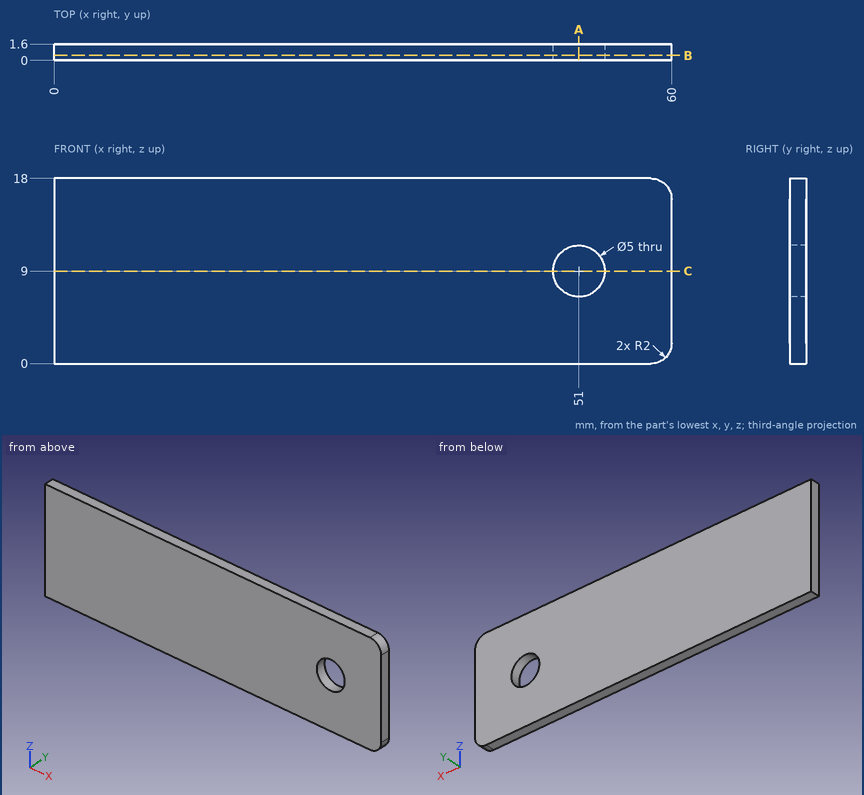
Can you work these out from the drawing? Everything is in mm from the part's minimum corner. Round coordinates to 2 decimals unless told otherwise and drop trailing zeros. Order: outer loops, then holes, each group sorted by start corner. A loop starts at its lowest first (then second) coordinate and runs counter-clockwise, first axis right, second up. Notation, with made-up numbers: (71, -25) -> (130, -25) arc R20 cw to (130, 9) -> close; hole circle Ø9 at (10, 71). An arc over 180 degrees is marked (long way). Return JSON: item names as keys, results as strings. Group by question number.
1. If we section it at B-B, the plane y = 0.5: Write out the boundary of the cut face in (x, z).
2. If we section it at A-A, the plane x = 51: Write out the boundary of the cut face in (y, z), then the cut area to 3 significant figures.
3. I need wall thicknesses on line 1 (X direction, y = 0.8, z = 8.75); line 2 (Z direction, x = 51, y = 0.7); line 3 (X direction, y = 0.95, z = 8). Which ranges of each line are inside material? Lowest first, please. Write a range as [from, to].
4. Will this pin go through, and if not, where does the flat tip stop? pin 1 (8 mm diameter, centred on x = 51, z = 9, fed in from +Y).
5. If we section it at C-C, the plane z = 9: Write out the boundary of the cut face in (x, y), then the cut area to 3 significant figures.
Output values:
{
 "1": {"outline": "(0, 0) -> (58, 0) arc R2 ccw to (60, 2) -> (60, 16) arc R2 ccw to (58, 18) -> (0, 18) -> close; hole circle Ø5 at (51, 9)"},
 "2": {"outline": "(0, 0) -> (1.6, 0) -> (1.6, 6.5) -> (0, 6.5) -> close; (0, 11.5) -> (1.6, 11.5) -> (1.6, 18) -> (0, 18) -> close", "area": "20.8 mm²"},
 "3": {"line 1": "[0, 48.51], [53.49, 60]", "line 2": "[0, 6.5], [11.5, 18]", "line 3": "[0, 48.71], [53.29, 60]"},
 "4": {"pin 1": "y = 1.6"},
 "5": {"outline": "(0, 0) -> (48.5, 0) -> (48.5, 1.6) -> (0, 1.6) -> close; (53.5, 0) -> (60, 0) -> (60, 1.6) -> (53.5, 1.6) -> close", "area": "88.0 mm²"}
}
